For this review, take the finished solid that the model builds, in its own axes (mm). Round coordinates to 2 decimals unless told otherwise and drop trailing zeros. Write each loop counter-clockwise with the first axis right and the second up, starting at its lowest first coordinate (ties: lowest second). Pieces come first, ordered by that corner, then holes. Notation, with made-up numbers: M 62,-18.75 L 71,-18.75 A25 ccw 71,18.25 Z; hole C -1.75,47 d3. An arc over 180 degrees is marked long. Answer in a Markdown table with one row per item.
Autodesk Inventor part; units mm, degrees
ref_plane "YZ Plane" through (0, 0, 0) normal (1, 0, 0) x (0, 1, 0)
ref_plane "XZ Plane" through (0, 0, 0) normal (0, 1, 0) x (-1, 0, 0)
ref_plane "XY Plane" through (0, 0, 0) normal (0, 0, 1) x (1, 0, 0)
sketch "Esboço1" plane through (0, 0, 0) normal (0, 0, 1) x (1, 0, 0)
  arc A0 (-32.6171, 0.9719) -> (-32.6171, -0.9719) centre (-32.3816, 0) ccw
  line L0 (-6, 0) -> (-7, 0)
  arc A1 (-6.8571, 0.9897) -> (-5.7551, 1.6967) centre (-6.7143, 1.9795) ccw
  arc A2 (-5.7551, -1.6967) -> (-7.0345, -1.0321) centre (-6.7143, -1.9795) ccw
  arc A3 (-6.8571, 0.9897) -> (-32.6171, 0.9719) centre (-19.7001, -52.3443) ccw
  arc A4 (-32.6171, -0.9719) -> (-7.0345, -1.0321) centre (-19.7001, 52.3443) ccw
  arc A5 (0, 2.5) -> (0, -2.5) centre (0, 0) ccw
  arc A6 (32.6171, -0.9719) -> (32.6171, 0.9719) centre (32.3816, 0) ccw
  line L1 (6, 0) -> (7, 0)
  arc A7 (5.7551, 1.6967) -> (6.8571, 0.9897) centre (6.7143, 1.9795) ccw
  arc A8 (7.0345, -1.0321) -> (5.7551, -1.6967) centre (6.7143, -1.9795) ccw
  arc A9 (32.6171, 0.9719) -> (6.8571, 0.9897) centre (19.7001, -52.3443) ccw
  arc A10 (7.0345, -1.0321) -> (32.6171, -0.9719) centre (19.7001, 52.3443) ccw
  arc A11 (0, -2.5) -> (0, 2.5) centre (0, 0) ccw
  arc A12 (0, 6) -> (-5.7551, 1.6967) centre (0, 0) ccw
  arc A13 (-5.7551, -1.6967) -> (0, -6) centre (0, 0) ccw
  arc A14 (0, -6) -> (5.7551, -1.6967) centre (0, 0) ccw
  arc A15 (5.7551, 1.6967) -> (0, 6) centre (0, 0) ccw
  point P0 (-6.7143, 2.9795)
  point P1 (-6.7143, 0.9795)
  point P2 (-6.7143, -0.9795)
  point P3 (-6.7143, -2.9795)
  point P4 (6.7143, 2.9795)
  point P5 (6.7143, 0.9795)
  point P6 (6.7143, -0.9795)
  point P7 (6.7143, -2.9795)
extrude "Extrusão1" add sketch "Esboço1" along normal blind 3
properties part number "HELICE"
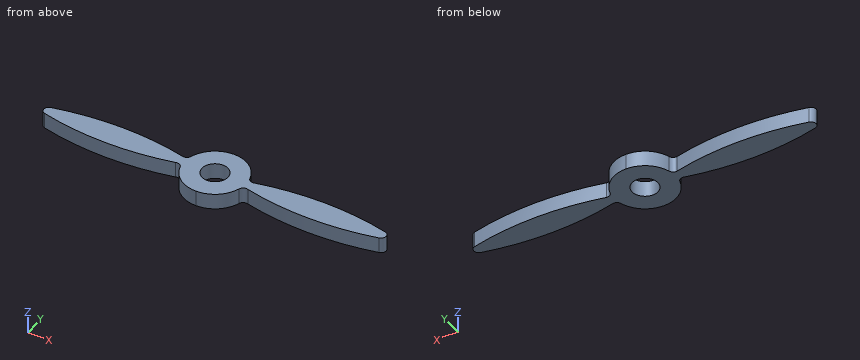
Q1. Take a section at D-D (y = -4.5). State the section outline as (x, z) points, then the cut area to 3 significant figures.
Found:
| item | result |
|---|---|
| outline | M -3.97,0 L 3.97,0 L 3.97,3 L -3.97,3 Z |
| area | 23.8 mm² |
Q2. For probe 1 along X at (y, z) = (0, 2.45); probe 2 along Y at (x, z) = (0, 1.75); probe 3 along Y at (x, z) = (-29, 2.85), list the stretches that pass through material, from the lowest coordinate up.
Found:
| item | result |
|---|---|
| probe 1 | -33.38 to -2.5, 2.5 to 33.38 |
| probe 2 | -6 to -2.5, 2.5 to 6 |
| probe 3 | -1.72 to 1.72 |
Q3. Take a section at A-A (y = 0). State the section outline as (x, z) points, then the cut area to 3 significant figures.
Found:
| item | result |
|---|---|
| outline | M -33.38,0 L -2.5,0 L -2.5,3 L -33.38,3 Z; M 2.5,0 L 33.38,0 L 33.38,3 L 2.5,3 Z |
| area | 185 mm² |
Q4. Insertion check: P1, Ø3, axis at x = -13.5, y = -2, coming from the -Z side; P2, Ø1.5, axis at y = -4, z = 0.5, coming from the -X side; P3, Ø1, axis at x = 23, z = 2, coming from the +Y side. Each pin has a flat end and moves straight along its axis. Give the tip position at first contact, or say it passes through.
Found:
| item | result |
|---|---|
| P1 | z = 0 |
| P2 | x = -5.04 |
| P3 | y = 2.44 |
Q5. Take a section at B-B (z = 1.5). State the section outline as (x, y) points.
Found:
| item | result |
|---|---|
| outline | M -32.62,-0.97 A54.86 ccw -7.03,-1.03 A1 cw -5.76,-1.7 A6 ccw 0,-6 A6 ccw 5.76,-1.7 A1 cw 7.03,-1.03 A54.86 ccw 32.62,-0.97 A1 ccw 32.62,0.97 A54.86 ccw 6.86,0.99 A1 cw 5.76,1.7 A6 ccw 0,6 A6 ccw -5.76,1.7 A1 cw -6.86,0.99 A54.86 ccw -32.62,0.97 A1 ccw Z; hole C 0,0 d5 |
Q6. Take a section at C-C (x = 3.5). State the section outline as (y, z) points, then the cut area to 3 significant figures.
Found:
| item | result |
|---|---|
| outline | M -4.87,0 L 4.87,0 L 4.87,3 L -4.87,3 Z |
| area | 29.2 mm² |
